from build123d import *

# Parameters (mm, degrees)
SKETCH1_R           = 11.75
SKETCH1_W           = 3.1
SKETCH1_H           = 5.1
BOSS_EXTRUDE1_DEPTH = 1.5


with BuildPart() as part:
    # Sketch1 (on Top Plane) → Boss-Extrude1 (new body)
    with BuildSketch(Plane(origin=(0, 0, 0), x_dir=(1, 0, 0), z_dir=(0, 1, 0))):
        with Locations(Location((0, 0, 0), (0, 0, 270))):
            Circle(SKETCH1_R)
        Rectangle(SKETCH1_W, SKETCH1_H, mode=Mode.SUBTRACT)
        Polygon((0.455975537, 4.338317439), (1.137082311, 10.81861552), (-1.137082311, 10.81861552), (-0.455975537, 4.338317439), align=None, mode=Mode.SUBTRACT)
        Polygon((2.081681544, 3.833682994), (5.190844864, 9.560049478), (3.089790717, 10.430334601), (1.239148612, 4.182671561), align=None, mode=Mode.SUBTRACT)
        Polygon((3.390522808, 2.745330804), (8.454400744, 6.845978303), (6.846323518, 8.454055528), (2.745676019, 3.390177592), align=None, mode=Mode.SUBTRACT)
        Polygon((4.183240111, 1.238952624), (10.430903151, 3.089594729), (9.560618028, 5.190648876), (3.834251544, 2.081485556), align=None, mode=Mode.SUBTRACT)
        Polygon((4.339149431, -0.456119123), (10.819447512, -1.137225897), (10.819447512, 1.136938725), (4.339149431, 0.455831951), align=None, mode=Mode.SUBTRACT)
        Polygon((3.834514986, -2.08182513), (9.56088147, -5.19098845), (10.431166593, -3.089934303), (4.183503553, -1.239292198), align=None, mode=Mode.SUBTRACT)
        Polygon((2.746162796, -3.390666394), (6.846810295, -8.45454433), (8.45488752, -6.846467104), (3.391009584, -2.745819606), align=None, mode=Mode.SUBTRACT)
        Polygon((1.239784616, -4.183383697), (3.090426721, -10.431046737), (5.191480868, -9.560761614), (2.082317548, -3.83439513), align=None, mode=Mode.SUBTRACT)
        Polygon((-0.455287131, -4.339293017), (-1.136393905, -10.819591098), (1.137770717, -10.819591098), (0.456663943, -4.339293017), align=None, mode=Mode.SUBTRACT)
        Polygon((-2.080993138, -3.834658572), (-5.190156458, -9.561025056), (-3.089102311, -10.431310179), (-1.238460206, -4.183647139), align=None, mode=Mode.SUBTRACT)
        Polygon((-3.389834402, -2.746306382), (-8.453712338, -6.846953881), (-6.845635112, -8.455031106), (-2.744987614, -3.39115317), align=None, mode=Mode.SUBTRACT)
        Polygon((-4.182551705, -1.239928202), (-10.430214745, -3.090570307), (-9.559929622, -5.191624454), (-3.833563138, -2.082461134), align=None, mode=Mode.SUBTRACT)
        Polygon((-4.338461025, 0.455143545), (-10.818759106, 1.136250319), (-10.818759106, -1.137914303), (-4.338461025, -0.456807529), align=None, mode=Mode.SUBTRACT)
        Polygon((-3.83382658, 2.080849552), (-9.560193064, 5.190012872), (-10.430478187, 3.088958725), (-4.182815147, 1.23831662), align=None, mode=Mode.SUBTRACT)
        Polygon((-2.74547439, 3.389690816), (-6.846121889, 8.453568752), (-8.454199114, 6.845491526), (-3.390321178, 2.744844027), align=None, mode=Mode.SUBTRACT)
        Polygon((-1.23909621, 4.182408119), (-3.089738315, 10.430071159), (-5.190792462, 9.559786036), (-2.081629142, 3.833419552), align=None, mode=Mode.SUBTRACT)
    extrude(amount=BOSS_EXTRUDE1_DEPTH)


solid = part.part
Can you work these out from the model? Positions are in its coordinate system, mm. Round coordinates to 2 decimals unless told otherwise and drop trailing zeros. Loops run counter-clockwise (first coordinate to the right, second up) from the corner with the lowest first, then second, coordinate; pieces in that order, holes last. Notation, with made-up numbers: (89, -35.75) - (118, -35.75) arc R32 cw to (118, -0.75) - close; hole circle Ø10 at (22, -7). An arc over 180 degrees is marked (long way). Answer in a Markdown table with one row per item. Add a question column.
Q1. I want a section at A-A on z = 0. List the corners of the cut face in (x, y) for me, and give its area (3 significant figures).
Q2. I want a section at B-B on x = 0. List the corners of the cut face in (y, z) for me.
Q3. I need wall thicknesses on L1, parallel to X at y = 0.4, z = 8.25; L2, parallel to Z at x = 10, y = 0.6; L3, parallel to X at y = 1.1, z = -6. Which ranges of each line are inside material? Lowest first, please.
Q4. I want a section at C-C on y = 0.55. Count the separate pieces of the cut face and the enclosed holes in it, and give its area (3 significant figures).
A:
| question | item | result |
|---|---|---|
| 1 | outline | (-11.75, 0) - (-10.82, 0) - (-10.82, 1.5) - (-11.75, 1.5) - close; (-4.34, 0) - (-1.55, 0) - (-1.55, 1.5) - (-4.34, 1.5) - close; (1.55, 0) - (4.34, 0) - (4.34, 1.5) - (1.55, 1.5) - close; (10.82, 0) - (11.75, 0) - (11.75, 1.5) - (10.82, 1.5) - close |
| 1 | area | 11.2 mm^2 |
| 2 | outline | (0, -11.75) - (1.5, -11.75) - (1.5, -10.82) - (0, -10.82) - close; (0, -4.34) - (1.5, -4.34) - (1.5, -2.55) - (0, -2.55) - close; (0, 2.55) - (1.5, 2.55) - (1.5, 4.34) - (0, 4.34) - close; (0, 10.82) - (1.5, 10.82) - (1.5, 11.75) - (0, 11.75) - close |
| 3 | L1 | -8.37 to -7.05, -6.68 to -4.48, -2.44 to -0.87, 0.87 to 2.44, 4.48 to 6.68, 7.05 to 8.37 |
| 3 | L2 | -6.17 to -4.13, -2.96 to -1.05, 1.05 to 2.96, 4.13 to 6.17 |
| 3 | L3 | -10.1 to -7.41, -4.86 to -3.26, -1.78 to -0.63, 0.63 to 1.78, 3.26 to 4.86, 7.41 to 10.1 |
| 4 | separate pieces | 1 |
| 4 | enclosed holes | 17 |
| 4 | area | 253 mm^2 |
